```python
from build123d import *

# Parameters (mm, degrees)
SKETCH1_R               = 6.35
BASIC_ROD_DEPTH         = 18.25625
BASIC_ROD_DEPTH_BACK    = 18.25625
THEX_DEPTH              = 18.25625
SKETCH2_R               = 2.11582
INTERNAL_CUT_DEPTH      = 19.25625
INTERNAL_CUT_DEPTH_BACK = 19.25625
SKETCH9_R               = 4
CUT_EXTRUDE1_DEPTH      = 19.99996
CUT_EXTRUDE2_REACH      = 14.7
SKETCH10_R              = 1.66624


with BuildPart() as part:
    # Sketch1 → Basic Rod (new body, two sides)
    with BuildSketch(Plane.XY) as basic_rod_sk:
        Circle(SKETCH1_R)
    extrude(amount=BASIC_ROD_DEPTH)
    extrude(basic_rod_sk.sketch, amount=-BASIC_ROD_DEPTH_BACK)

    # Sketch8 → THex (add, symmetric)
    with BuildSketch(Plane.XY):
        with BuildLine():
            Line((-0.888411378, 6.819423871), (-5.461588622, 4.179098758))
            ThreePointArc((-5.461588622, 4.179098758), (-5.955700003, 3.438525), (-6.35, 2.640325113))
            Line((-6.35, 2.640325113), (-6.35, -2.640325113))
            ThreePointArc((-6.35, -2.640325113), (-5.955700003, -3.438525), (-5.461588622, -4.179098758))
            Line((-5.461588622, -4.179098758), (-0.888411378, -6.819423871))
            ThreePointArc((-0.888411378, -6.819423871), (0, -6.87705), (0.888411378, -6.819423871))
            Line((0.888411378, -6.819423871), (5.461588622, -4.179098758))
            ThreePointArc((5.461588622, -4.179098758), (5.955700003, -3.438525), (6.35, -2.640325113))
            Line((6.35, -2.640325113), (6.35, 2.640325113))
            ThreePointArc((6.35, 2.640325113), (5.955700003, 3.438525), (5.461588622, 4.179098758))
            Line((5.461588622, 4.179098758), (0.888411378, 6.819423871))
            ThreePointArc((0.888411378, 6.819423871), (0, 6.87705), (-0.888411378, 6.819423871))
        make_face()
    extrude(amount=THEX_DEPTH, both=True)

    # Sketch2 → Internal Cut (cut, two sides)
    with BuildSketch(Plane.XY) as internal_cut_sk:
        Circle(SKETCH2_R)
    extrude(amount=INTERNAL_CUT_DEPTH, mode=Mode.SUBTRACT)
    extrude(internal_cut_sk.sketch, amount=-INTERNAL_CUT_DEPTH_BACK, mode=Mode.SUBTRACT)

    # Sketch9 → Cut-Extrude1 (cut)
    with BuildSketch(Plane.XY.offset(18.25625)):
        Circle(SKETCH9_R)
    extrude(amount=-CUT_EXTRUDE1_DEPTH, mode=Mode.SUBTRACT)

    # Sketch10 → Cut-Extrude2 (cut, up to next)
    with BuildSketch(Plane.ZY.offset(6.35), mode=Mode.PRIVATE) as cut_extrude2_sk1:
        with Locations((5.25399, 0)):
            Circle(SKETCH10_R)
    cut_extrude2_tool1 = extrude(cut_extrude2_sk1.sketch, amount=-CUT_EXTRUDE2_REACH, mode=Mode.PRIVATE) & part.part
    add(cut_extrude2_tool1.solids().sort_by_distance((-6.35, 0, 5.25399))[0], mode=Mode.SUBTRACT)
    # Sketch10 → Cut-Extrude2 (cut, up to next)
    with BuildSketch(Plane.ZY.offset(6.35), mode=Mode.PRIVATE) as cut_extrude2_sk2:
        with Locations((13.25499, 0)):
            Circle(SKETCH10_R)
    cut_extrude2_tool2 = extrude(cut_extrude2_sk2.sketch, amount=-CUT_EXTRUDE2_REACH, mode=Mode.PRIVATE) & part.part
    add(cut_extrude2_tool2.solids().sort_by_distance((-6.35, 0, 13.25499))[0], mode=Mode.SUBTRACT)


solid = part.part
```
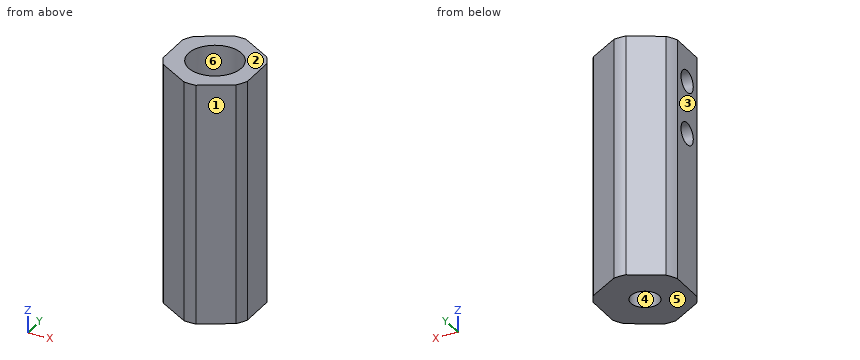
The listing builds one solid part. Answer for the finished solid, in the listing's coordinates (mm). Face numbers are marked on the shaded views. A direction names the side the tool comes from. Give positions to 0.01 mm unless a question says otherwise; leave off trailing zeros. Loops run counter-clockwise (first coordinate to the right, second up) from the corner with the lowest first, then second, coordinate; pieces in that order, holes last. Notation, with made-up numbers: (57.25, 57) - (61.25, 57) arc R19 cw to (61.25, 91) - close; hole circle Ø3 at (16.25, 36). An arc over 180 degrees is marked (long way). Return JSON: item names as keys, results as strings. Group by question number.
1. Find section D-D (z = -15). Write down the section's boundary in (x, y), then the cut area to 3 significant figures.
2. Determine the mould class of the marked faces 1, 2, 3 and 4 for opening direction X: pulls with the +X half, pulls with the -X half, needs draft (parallel to the pull), parting line crosses it, or undercut.
3. Straight lines are drawn through the part: line 1 (Z direction, x = -4.15, y = 0); line 2 (Z direction, x = -5.25, y = 1); line 3 (Y direction, x = 0, z = 3.25). For each, find the intervals that lie inside material, in ascending order. Write a range as [from, to].
4. Find section B-B (y = 0). Write down the section's boundary in (x, z).
5. Find section A-A (z = 11). Write down the section's boundary in (x, y), then the cut area to 3 significant figures.
6. Which of the six approach directions +Z, -Z, +X, -X, +Y, -Y give full straight-line access (tool end or side, diameter ignored) to the marked faces 5 and 6?
7. Given pin 1 Ø8 at (y, z) = (-5.5, -4.5) entering from -X; pin 2 Ø4 at (x, z) = (4, 9.5) entering from +Y; pin 3 Ø3 at (y, z) = (0, 5.25) entering from -X; pin 4 Ø4 at (x, y) = (0, 0.5) entering from +Z, each flat-ended and moving along its own axis, determine where each tip first touches the part or whether it passes through.
8. Find section C-C (x = 0). Write down the section's boundary in (y, z), then the cut area to 3 significant figures.
Verdict:
{
 "1": {"outline": "(-6.35, -2.64) arc R6.88 ccw to (-5.46, -4.18) - (-0.89, -6.82) arc R6.88 ccw to (0.89, -6.82) - (5.46, -4.18) arc R6.88 ccw to (6.35, -2.64) - (6.35, 2.64) arc R6.88 ccw to (5.46, 4.18) - (0.89, 6.82) arc R6.88 ccw to (-0.89, 6.82) - (-5.46, 4.18) arc R6.88 ccw to (-6.35, 2.64) - close; hole circle Ø4.23 at (0, 0)", "area": "123 mm^2"},
 "2": {"face 1": "pulls with the +X half", "face 2": "needs draft", "face 3": "pulls with the -X half", "face 4": "undercut"},
 "3": {"line 1": "z = [-18.26, 3.59], [6.92, 11.59], [14.92, 18.26]", "line 2": "z = [-18.26, 3.92], [6.59, 11.92], [14.59, 18.26]", "line 3": "y = [-6.88, -4], [4, 6.88]"},
 "4": {"outline": "(-6.35, -18.26) - (-2.12, -18.26) - (-2.12, -1.74) - (-4, -1.74) - (-4, 3.59) - (-6.35, 3.59) - close; (-6.35, 6.92) - (-4, 6.92) - (-4, 11.59) - (-6.35, 11.59) - close; (-6.35, 14.92) - (-4, 14.92) - (-4, 18.26) - (-6.35, 18.26) - close; (2.12, -18.26) - (6.35, -18.26) - (6.35, 18.26) - (4, 18.26) - (4, -1.74) - (2.12, -1.74) - close"},
 "5": {"outline": "(-6.35, -2.64) arc R6.88 ccw to (-5.46, -4.18) - (-0.89, -6.82) arc R6.88 ccw to (0.89, -6.82) - (5.46, -4.18) arc R6.88 ccw to (6.35, -2.64) - (6.35, 2.64) arc R6.88 ccw to (5.46, 4.18) - (0.89, 6.82) arc R6.88 ccw to (-0.89, 6.82) - (-5.46, 4.18) arc R6.88 ccw to (-6.35, 2.64) - close; hole circle Ø8 at (0, 0)", "area": "87.1 mm^2"},
 "6": {"face 5": "-Z, +X, -X, +Y, -Y", "face 6": "+Z"},
 "7": {"pin 1": "stops at x = -6.35", "pin 2": "stops at y = 6.18", "pin 3": "stops at x = 3.71", "pin 4": "stops at z = -1.74"},
 "8": {"outline": "(-6.88, -18.26) - (-2.12, -18.26) - (-2.12, -1.74) - (-4, -1.74) - (-4, 18.26) - (-6.88, 18.26) - close; (2.12, -18.26) - (6.88, -18.26) - (6.88, 18.26) - (4, 18.26) - (4, -1.74) - (2.12, -1.74) - close", "area": "272 mm^2"}
}
